CAD build for the part. Positions are in the model's coordinates, mm. A direction names the side the tool comes from. Round coordinates to 2 decimals unless told otherwise and drop trailing zeros. Loops run counter-clockwise (first coordinate to the right, second up) from the corner with the lowest first, then second, coordinate; pieces in that order, holes last. Notation, with made-up numbers: (-5, 26) - (49, 26) arc R21 cw to (49, 39) - close; hole circle Ø6 at (-33.75, 2.25). An arc over 180 degrees is marked (long way). One line per question, with ' | ' between items.
```python
from build123d import *

# Parameters (mm, degrees)
SKETCH1_W               = 60
SKETCH1_H               = 250
BOSS_EXTRUDE1_DEPTH     = 16
CHAMFER2_SIZE           = 1
SKETCH2_R               = 2
CUT_EXTRUDE1_DEPTH      = 15
SKETCH3_W               = 45
SKETCH3_H               = 50
CUT_EXTRUDE2_DEPTH      = 258.596583828
CUT_EXTRUDE3_DEPTH      = 256.953609078
CUT_EXTRUDE3_DEPTH_BACK = 256.953609078
SKETCH4_R               = 4
SKETCH5_W               = 60
SKETCH5_H               = 25
CUT_EXTRUDE4_DEPTH      = 258.596583828
ESBO_O1_W               = 45
ESBO_O1_H               = 33
CORTE_EXTRUS_O1_DEPTH   = 234.411653522
FILETE1_R               = 25


with BuildPart() as part:
    # Sketch1 → Boss-Extrude1 (new body)
    with BuildSketch(Plane.XY):
        with Locations((30, 125)):
            Rectangle(SKETCH1_W, SKETCH1_H)
    extrude(amount=BOSS_EXTRUDE1_DEPTH)

    # Chamfer2
    chamfer2_edges = [part.edges().sort_by_distance(p)[0] for p in [
        (30, 0, 16),
    ]]
    chamfer(chamfer2_edges, length=CHAMFER2_SIZE)

    # Sketch2 → Cut-Extrude1 (cut)
    with BuildSketch(Plane(origin=(0, 0, 0), x_dir=(-1, 0, 0), z_dir=(0, -1, 0))):
        with Locations(Location((-41.5, -7.5, 0), (0, 0, 90))):
            Circle(SKETCH2_R)
        with Locations(Location((-18.5, -7.5, 0), (0, 0, 90))):
            Circle(SKETCH2_R)
    extrude(amount=-CUT_EXTRUDE1_DEPTH, mode=Mode.SUBTRACT)

    # Sketch3 → Cut-Extrude2 (cut, through all)
    with BuildSketch(Plane(origin=(0, 0, 0), x_dir=(-1, 0, 0), z_dir=(0, 0, -1))):
        with Locations((-30, 200)):
            Rectangle(SKETCH3_W, SKETCH3_H)
    extrude(amount=-CUT_EXTRUDE2_DEPTH, mode=Mode.SUBTRACT)

    # Sketch4 → Cut-Extrude3 (cut, two sides: drawn at the far end of the back side and taken through both)
    with BuildSketch(Plane.ZY.offset(-52.5).offset(-CUT_EXTRUDE3_DEPTH_BACK)):
        with Locations((8, 200)):
            Circle(SKETCH4_R)
    extrude(amount=CUT_EXTRUDE3_DEPTH + CUT_EXTRUDE3_DEPTH_BACK, mode=Mode.SUBTRACT)

    # Sketch5 → Cut-Extrude4 (cut, through all)
    with BuildSketch(Plane(origin=(0, 0, 0), x_dir=(-1, 0, 0), z_dir=(0, 0, -1))):
        with Locations((-30, 237.5)):
            Rectangle(SKETCH5_W, SKETCH5_H)
    extrude(amount=-CUT_EXTRUDE4_DEPTH, mode=Mode.SUBTRACT)

    # Esboço1 → Corte-extrusão1 (cut, through all)
    with BuildSketch(Plane(origin=(0, 0, 0), x_dir=(-1, 0, 0), z_dir=(0, 0, -1))):
        with Locations((-30, 158.5)):
            Rectangle(ESBO_O1_W, ESBO_O1_H)
    extrude(amount=-CORTE_EXTRUS_O1_DEPTH, mode=Mode.SUBTRACT)

    # Filete1
    # the kernel refuses this fillet: 25 mm, written as the material it takes off along each edge
    with BuildSketch(Plane(origin=(-5.809518948, 225, 0), x_dir=(0, 0, 1), z_dir=(1, 0, 0)), Plane(origin=(-58.309518948, 225, 0), x_dir=(0, 0, 1), z_dir=(1, 0, 0))) as filete1_piece_1:
        with BuildLine():
            CenterArc((25, 23.323807579), FILETE1_R, 180, 68.899803976)
            Line((0, 23.323807579), (-0.5, 23.323807579))
            Line((-0.5, 23.323807579), (-0.5, 0))
            Line((-0.5, 0), (0, -0.5))
            ThreePointArc((0, -0.5), (8, -0.5), (15.82, -0.466476152))
            Line((15.82, -0.466476152), (16, 0))
        make_face()
    extrude(amount=124.119037897, mode=Mode.SUBTRACT)


solid = part.part
```
(1) Cut at B-B, the plane x = 18.5. Write the cut outline in (y, z).
Results found:
outline: (0, 0) - (142, 0) - (142, 16) - (1, 16) - (0, 15) - (0, 9.5) - (15, 9.5) - (15, 5.5) - (0, 5.5) - close
(2) Cut at A-A, the plane z = 7.5. Write the cut outline in (x, y).
Results found:
outline: (0, 0) - (16.5, 0) - (16.5, 15) - (20.5, 15) - (20.5, 0) - (39.5, 0) - (39.5, 15) - (43.5, 15) - (43.5, 0) - (60, 0) - (60, 196.03) - (52.5, 196.03) - (52.5, 142) - (7.5, 142) - (7.5, 196.03) - (0, 196.03) - close; (0, 203.97) - (7.5, 203.97) - (7.5, 219.53) - (0, 219.53) - close; (52.5, 203.97) - (60, 203.97) - (60, 219.53) - (52.5, 219.53) - close
(3) Tool access for faces 1 (the face through (7.5, 183, 8)), 2 (the face through (19, 15, 8)), 3 (the face through (60, 111, 8)): list every direction of +Z, -Z, +X, -X, +Y, -Y with a clear straight run to the whole face (end or side of a thin tool).
Results found:
face 1: +Z, -Z, +Y | face 2: -Y | face 3: +Z, -Z, +X, +Y, -Y
(4) Probe L1, parallel to X at y = 6, z = 7.5; L2, parallel to X at y = 159.5, z = 14.5; L3, parallel to Z at x = 58.25, y = 200. List the from-to ranges inside material, lowest first.
Results found:
L1: x = 0 to 16.5, 20.5 to 39.5, 43.5 to 60 | L2: x = 0 to 7.5, 52.5 to 60 | L3: z = 0 to 4, 12 to 16
(5) Drop flat-ended pins along their axis: P1, Ø6.5, axis at x = 41.5, z = 7.5, coming from the +Y side; P2, Ø4.5, axis at x = 18.5, z = 7.5, coming from the -Y side; P3, Ø1.5, axis at x = 52, z = 9.5, coming from the +Y side. Give the stop position or say it passes through.
Results found:
P1: stops at y = 142 | P2: stops at y = 0 | P3: stops at y = 221.72
(6) Two-plate mould, pull along Z, no slides. Class faces 4 (the face through (42, 15, 8)), 5 (the face through (30, 0, 7)), 6 (the face through (3.698, 215.644, 4.266)), 7 (the face through (56.303, 203.966, 7.479)): released by +Z, released by -Z, zero draft, split by the parting line, or undercut.
Results found:
face 4: undercut | face 5: zero draft | face 6: released by -Z | face 7: undercut
